```python
from build123d import *

# Parameters (mm, degrees)
RESSALTO_EXTRUS_O1_DEPTH = 10
CORTE_EXTRUS_O1_DEPTH    = 29.722813233


with BuildPart() as part:
    # Esboço1 → Ressalto-extrusão1 (new body)
    with BuildSketch(Plane(origin=(0, 0, 0), x_dir=(1, 0, 0), z_dir=(0, 1, 0))):
        with BuildLine():
            Line((-7.5, 20.68211788), (-7.5, 25))
            Line((-7.5, 25), (7.5, 25))
            Line((7.5, 25), (7.5, 20.68211788))
            ThreePointArc((7.5, 20.68211788), (8.766838517, 20.177773475), (10, 19.595917942))
            Line((10, 19.595917942), (10, -19.595917942))
            ThreePointArc((10, -19.595917942), (8.766838517, -20.177773475), (7.5, -20.68211788))
            Line((7.5, -20.68211788), (7.5, -25))
            Line((7.5, -25), (-7.5, -25))
            Line((-7.5, -25), (-7.5, -20.68211788))
            ThreePointArc((-7.5, -20.68211788), (-8.766838517, -20.177773475), (-10, -19.595917942))
            Line((-10, -19.595917942), (-10, 19.595917942))
            ThreePointArc((-10, 19.595917942), (-8.766838517, 20.177773475), (-7.5, 20.68211788))
        make_face()
    extrude(amount=RESSALTO_EXTRUS_O1_DEPTH)

    # Esboço2 → Corte-extrusão1 (cut, through all)
    with BuildSketch(Plane(origin=(0, 10, 0), x_dir=(1, 0, 0), z_dir=(0, 1, 0))):
        with BuildLine():
            Line((5.25, 16.5), (-5.25, 16.5))
            ThreePointArc((-5.25, 16.5), (-6.957106781, 17.207106781), (-6.25, 15.5))
            Line((-6.25, 15.5), (-6.25, -5.25))
            ThreePointArc((-6.25, -5.25), (-6.957106781, -6.957106781), (-5.25, -6.25))
            Line((-5.25, -6.25), (5.25, -6.25))
            ThreePointArc((5.25, -6.25), (6.957106781, -6.957106781), (6.25, -5.25))
            Line((6.25, -5.25), (6.25, 15.5))
            ThreePointArc((6.25, 15.5), (6.957106781, 17.207106781), (5.25, 16.5))
        make_face()
    extrude(amount=-CORTE_EXTRUS_O1_DEPTH, mode=Mode.SUBTRACT)


solid = part.part
```
The listing builds one solid part. Answer for the finished solid, in the listing's coordinates (mm). A direction names the side the tool comes from. Coordinates: 2 decimals unless noted, no trailing zeros. Loops run counter-clockwise (first coordinate to the right, second up) from the corner with the lowest first, then second, coordinate; pieces in that order, holes last. Notation, with made-up numbers: (85, 62.25) - (111, 62.25) arc R27 ccw to (111, 101.25) - close; hole circle Ø5 at (80.25, 31). An arc over 180 degrees is marked (long way). Use a Markdown table: item, result. Add a question column.
1) Given pin 1 (1.3 mm diameter, centred on y = 5.5, z = -22, fed in from -X); pin 2 (2 mm diameter, centred on y = 3.5, z = 24, fed in from +X); pin 3 (4.5 mm diameter, centred on y = 2.5, z = -22, fed in from +X), each flat-ended and moving along its own axis, determine where each tip first touches the part or whether it passes through.
2) The part is cut by section A-A, the plane z = -12. Give the vertices of the cut face in (x, y).
3) The mould has two halves that part along X. Classify faces 6 (the cylindrical face through (6.98, 5.07, -17.183)), 7 (the flat face through (0, 5, -25)), 8 (the cylindrical face through (-8.78, 4.93, -20.17)): released by +X, released by -X, zero draft, split by the parting line, or undercut.
4) The part is cut by section C-C, the plane y = 5. Give the vertices of the cut face in (x, z).
5) For faces 1 (the cylindrical face through (8.78, 4.93, 20.17)), 2 (the flat face through (7.5, 5, -23)), 3 (the flat face through (-7.5, 5, 23)), 4 (the flat face through (-7.5, 5, -23)), 5 (the flat face through (0, 5, -16.5)), determine the directions among +Z, -Z, +X, -X, +Y, -Y from which every point of the face is accessible in a straight line to the end or side of a thin tool.
6) The part is cut by section B-B, the plane x = -2.75. Give the vertices of the cut face in (y, z).
7) Find the intervals of material crossed by line 1 (Z direction, x = -3, y = 7.75); line 2 (X direction, y = 4.5, z = 1); line 3 (X direction, y = 4.5, z = 7), in increasing order.
Here are the results:
| question | item | result |
|---|---|---|
| 1 | pin 1 | stops at x = -7.5 |
| 1 | pin 2 | stops at x = 7.5 |
| 1 | pin 3 | stops at x = 9.69 |
| 2 | outline | (-10, 0) - (-6.25, 0) - (-6.25, 10) - (-10, 10) - close; (6.25, 0) - (10, 0) - (10, 10) - (6.25, 10) - close |
| 3 | face 6 | undercut |
| 3 | face 7 | zero draft |
| 3 | face 8 | released by -X |
| 4 | outline | (-10, -19.6) arc R22 ccw to (-7.5, -20.68) - (-7.5, -25) - (7.5, -25) - (7.5, -20.68) arc R22 ccw to (10, -19.6) - (10, 19.6) arc R22 ccw to (7.5, 20.68) - (7.5, 25) - (-7.5, 25) - (-7.5, 20.68) arc R22 ccw to (-10, 19.6) - close; hole (-6.25, -15.5) arc R1 ccw (long way) to (-5.25, -16.5) - (5.25, -16.5) arc R1 ccw (long way) to (6.25, -15.5) - (6.25, 5.25) arc R1 ccw (long way) to (5.25, 6.25) - (-5.25, 6.25) arc R1 ccw (long way) to (-6.25, 5.25) - close |
| 5 | face 1 | +Z, +X, +Y, -Y |
| 5 | face 2 | -Z, +X, +Y, -Y |
| 5 | face 3 | +Z, -X, +Y, -Y |
| 5 | face 4 | -Z, -X, +Y, -Y |
| 5 | face 5 | +Y, -Y |
| 6 | outline | (0, -25) - (10, -25) - (10, -16.5) - (0, -16.5) - close; (0, 6.25) - (10, 6.25) - (10, 25) - (0, 25) - close |
| 7 | line 1 | z = -25 to -16.5, 6.25 to 25 |
| 7 | line 2 | x = -10 to -6.25, 6.25 to 10 |
| 7 | line 3 | x = -10 to -6.91, -5.59 to 5.59, 6.91 to 10 |
